from build123d import *

# Parameters (mm, degrees)
SKETCH2_W               = 28.702
SKETCH2_H               = 12.7
BOSS_EXTRUDE1_DEPTH     = 12.7
CUT_EXTRUDE1_DEPTH      = 34.858304801
CUT_EXTRUDE1_DEPTH_BACK = 34.858304801
SKETCH3_R               = 2.286
FILLET1_R               = 2.54
SKETCH4_W               = 19.05
SKETCH4_H               = 19.05
BOSS_EXTRUDE2_DEPTH     = 3.175
FILLET2_R               = 0.508
FILLET3_R               = 1.27


with BuildPart() as part:
    # Sketch2 → Boss-Extrude1 (new body)
    with BuildSketch(Plane.XY):
        with Locations((-14.351, -6.35)):
            Rectangle(SKETCH2_W, SKETCH2_H)
    extrude(amount=BOSS_EXTRUDE1_DEPTH)

    # Sketch3 → Cut-Extrude1 (cut, two sides: drawn at the far end of the back side and taken through both)
    with BuildSketch(Plane.XY.offset(12.7).offset(-CUT_EXTRUDE1_DEPTH_BACK)):
        with Locations((-6.35, -6.35)):
            Circle(SKETCH3_R)
    extrude(amount=CUT_EXTRUDE1_DEPTH + CUT_EXTRUDE1_DEPTH_BACK, mode=Mode.SUBTRACT)

    # Fillet1
    fillet1_edges = [part.edges().sort_by_distance(p)[0] for p in [
        (0, -12.7, 6.35),
        (0, 0, 6.35),
    ]]
    fillet(fillet1_edges, radius=FILLET1_R)

    # Sketch4 → Boss-Extrude2 (add)
    with BuildSketch(Plane.ZY.offset(28.702)):
        with Locations((6.35, -6.35)):
            Rectangle(SKETCH4_W, SKETCH4_H)
    extrude(amount=-BOSS_EXTRUDE2_DEPTH)

    # Fillet2
    fillet2_edges = [part.edges().sort_by_distance(p)[0] for p in [
        (0, -6.35, 0),
        (0, -6.35, 12.7),
        (-14.0335, 0, 0),
        (-0.743948776, -0.743948776, 0),
        (-0.743948776, -11.956051224, 0),
        (-14.0335, 0, 12.7),
        (-0.743948776, -0.743948776, 12.7),
        (-0.743948776, -11.956051224, 12.7),
        (-14.0335, -12.7, 0),
        (-14.0335, -12.7, 12.7),
    ]]
    fillet(fillet2_edges, radius=FILLET2_R)

    # Fillet3
    fillet3_edges = [part.edges().sort_by_distance(p)[0] for p in [
        (-27.1145, 3.175, 15.875),
        (-27.1145, -15.875, 15.875),
        (-27.1145, -15.875, -3.175),
        (-27.1145, 3.175, -3.175),
    ]]
    fillet(fillet3_edges, radius=FILLET3_R)


solid = part.part
Design review of the part built by this model. Coordinates are the model's own, in mm. A direction names the side the tool comes from. Give positions to 0.01 mm unless a question says otherwise; leave off trailing zeros. Write each loop counter-clockwise with the first axis right and the second up, starting at its lowest first coordinate (ties: lowest second). Pieces come first, ordered by that corner, then holes. Notation, with made-up numbers: M -25.5,78.5 L -8.5,78.5 A25 cw -8.5,115.5 Z; hole C -38.5,-28 d10. An arc over 180 degrees is marked long. Answer as a JSON object with one key per item and string values. Group by question number.
1) Mouldability with a two-part tool opening along X and no side actions: class faces 6 (the face through (-27.092, -15.493, -2.813)), 7 (the face through (-0.764, -11.976, 6.432)), 8 (the face through (-8.164, -7.741, 6.261)) as released by +X, released by -X, zero draft, split by the parting line, or undercut.
2) We need section A-A (y = -6.35). Give the boundary of the cut face in (x, z) (3 decimals), and give its area (3 significant figures).
3) For line 1 along X through (y, z) = (-6.35, 3); line 2 along Y through (x, z) = (-6.35, 5); line 3 along Z through (x, y) = (-4.25, -8.25), list the stretches that pass through material, from the lowest coordinate up.
4) We need section B-B (x = -6.35). Give the boundary of the cut face in (y, z).
5) Tool access review of faces 1 (the face through (-13, -6, 12.7)), 2 (the face through (-14, -12.7, 6)), 3 (the face through (-28.702, -6, 6)), 4 (the face through (-14, 0, 6)), 5 (the face through (-13, -6, 0)): name each direction out of +Z, -Z, +X, -X, +Y, -Y from which nothing blocks a thin tool from reaching the whole face with its end or side.
6) We need section D-D (x = -10.75). Give the boundary of the cut face in (y, z).
7) Clearance check with flat-ended pins moving along their axes: pin 1 Ø6 at (x, y) = (-6.35, -6.35) entering from -Z; pin 2 Ø2 at (x, z) = (-12, 11) entering from -Y; pin 3 Ø3 at (x, z) = (-16, 1) entering from +Y. State where each tip first meets the part, or that it passes through.
8) We need section C-C (z = 7.75). Give the boundary of the cut face in (x, y) (3 decimals).
Answer key:
{
 "1": {"face 6": "zero draft", "face 7": "released by +X", "face 8": "undercut"},
 "2": {"outline": "M -28.702,-3.175 L -25.527,-3.175 L -25.527,0 L -8.636,0 L -8.636,12.7 L -25.527,12.7 L -25.527,15.875 L -28.702,15.875 Z; M -4.064,0 L -0.508,0 A0.508 ccw 0,0.508 L 0,12.192 A0.508 ccw -0.508,12.7 L -4.064,12.7 Z", "area": "327 mm²"},
 "3": {"line 1": "x = -28.7 to -8.64, -4.06 to 0", "line 2": "y = -12.7 to -8.64, -4.06 to 0", "line 3": "z = 0 to 12.7"},
 "4": {"outline": "M -12.7,0.51 A0.51 ccw -12.19,0 L -8.64,0 L -8.64,12.7 L -12.19,12.7 A0.51 ccw -12.7,12.19 Z; M -4.06,0 L -0.51,0 A0.51 ccw 0,0.51 L 0,12.19 A0.51 ccw -0.51,12.7 L -4.06,12.7 Z"},
 "5": {"face 1": "+Z, +X, +Y, -Y", "face 2": "+Z, -Z, +X, -Y", "face 3": "+Z, -Z, -X, +Y, -Y", "face 4": "+Z, -Z, +X, +Y", "face 5": "-Z, +X, +Y, -Y"},
 "6": {"outline": "M -12.7,0.51 A0.51 ccw -12.19,0 L -0.51,0 A0.51 ccw 0,0.51 L 0,12.19 A0.51 ccw -0.51,12.7 L -12.19,12.7 A0.51 ccw -12.7,12.19 Z"},
 "7": {"pin 1": "stops at z = 0", "pin 2": "stops at y = -12.7", "pin 3": "stops at y = 0"},
 "8": {"outline": "M -28.702,-15.875 L -25.527,-15.875 L -25.527,-12.7 L -2.54,-12.7 A2.54 ccw 0,-10.16 L 0,-2.54 A2.54 ccw -2.54,0 L -25.527,0 L -25.527,3.175 L -28.702,3.175 Z; hole C -6.35,-6.35 d4.572"}
}
